Read the model definition and answer for the solid it produces. Units are mm, in the model's axes. Coordinates: 2 decimals unless noted, no trailing zeros. Order: outer loops, then holes, each group sorted by start corner. A loop starts at its lowest first (then second) coordinate and runs counter-clockwise, first axis right, second up. Notation, with made-up numbers: M 28,13.25 L 61,13.25 A38 ccw 61,52.25 Z; hole C 41,-33.75 d5. An arc over 180 degrees is marked long. One line per question, with ' | ' between items. Start each with the question number.
1) Find section C-C, the plane z = 0. Write down the section's boundary in (x, y).
2) Find section B-B, the plane y = 0.6. Write down the section's boundary in (x, z).
3) Given P1, Ø2, axis at y = 1, z = 5, coming from the +X side; P2, Ø12.5, axis at x = -24.5, z = -2, coming from the +Y side; P3, Ø2, axis at x = -29, z = -5, coming from the -Y side; P4, Ø0.6, axis at x = -2, y = 2.5, coming from the -Z side, each flat-ended and moving along its own axis, determine where each tip first touches the part or whether it passes through.
4) Consider probe 1 along Z at (x, y) = (-26, 0.65); probe 2 along Y at (x, z) = (-35, 6); probe 3 along X at (y, z) = (2.9, 1.75). Determine where each line is inside the solid, lowest interval first.
5) Find section A-A, the plane x = -25.5. Write down the section's boundary in (y, z), plus the area to 3 significant figures.
6) Find section D-D, the plane z = 7. Write down the section's boundary in (x, y), plus the area to 3 significant figures.
from build123d import *

# Parameters (mm, degrees)
SZKIC1_R                    = 1.5
DODANIE_WYCI_GNI_CIE1_DEPTH = 1.5
SZKIC2_W                    = 10.5
SZKIC2_H                    = 5.6
DODANIE_WYCI_GNI_CIE2_DEPTH = 1.86


with BuildPart() as part:
    # Szkic1 → Dodanie-wyciągnięcie1 (new body)
    with BuildSketch(Plane(origin=(0, 0, 0), x_dir=(1, 0, 0), z_dir=(0, 1, 0))):
        with BuildLine():
            Line((-39.2, 12.5), (0, 12.5))
            ThreePointArc((0, 12.5), (12.5, 0), (0, -12.5))
            Line((0, -12.5), (-39.2, -12.5))
            Line((-39.2, -12.5), (-39.2, 12.5))
        make_face()
        with Locations(Location((-25.5, 8, 0), (0, 0, 270))):
            Circle(SZKIC1_R, mode=Mode.SUBTRACT)
        with Locations(Location((-25.5, -8, 0), (0, 0, 90))):
            Circle(SZKIC1_R, mode=Mode.SUBTRACT)
    extrude(amount=DODANIE_WYCI_GNI_CIE1_DEPTH)

    # Szkic2 → Dodanie-wyciągnięcie2 (add)
    with BuildSketch(Plane(origin=(0, 1.5, 0), x_dir=(1, 0, 0), z_dir=(0, 1, 0))):
        Rectangle(SZKIC2_W, SZKIC2_H)
    extrude(amount=DODANIE_WYCI_GNI_CIE2_DEPTH)


solid = part.part
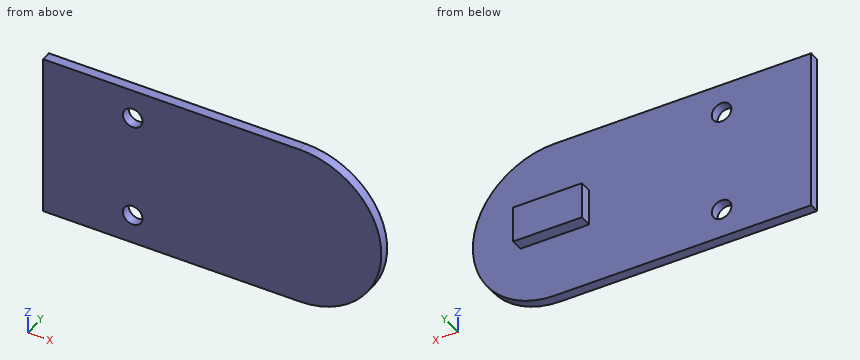
Report:
1) outline: M -39.2,0 L 12.5,0 L 12.5,1.5 L 5.25,1.5 L 5.25,3.36 L -5.25,3.36 L -5.25,1.5 L -39.2,1.5 Z
2) outline: M -39.2,-12.5 L 0,-12.5 A12.5 ccw 0,12.5 L -39.2,12.5 Z; hole C -25.5,-8 d3; hole C -25.5,8 d3
3) P1: stops at x = 11.84 | P2: stops at y = 1.5 | P3: stops at y = 0 | P4: stops at z = -2.8
4) probe 1: z = -12.5 to -9.41, -6.59 to 6.59, 9.41 to 12.5 | probe 2: y = 0 to 1.5 | probe 3: x = -5.25 to 5.25
5) outline: M 0,-12.5 L 1.5,-12.5 L 1.5,-9.5 L 0,-9.5 Z; M 0,-6.5 L 1.5,-6.5 L 1.5,6.5 L 0,6.5 Z; M 0,9.5 L 1.5,9.5 L 1.5,12.5 L 0,12.5 Z | area: 28.5 mm^2
6) outline: M -39.2,0 L -26.62,0 L -26.62,1.5 L -39.2,1.5 Z; M -24.38,0 L 10.36,0 L 10.36,1.5 L -24.38,1.5 Z | area: 71.0 mm^2
